from build123d import *

# Parameters (mm, degrees)
EXTRUDE_1_DEPTH     = 40
EXTRUDE_START       = 1
EXTRUDE_2_DEPTH     = 1
CUT_EXTRUDE_7_REACH = 83
FILLET_1_R          = 3
EXTRUDE_6_DEPTH     = 41
SKETCH_2_W          = 15.763743406
SKETCH_2_H          = 16
CUT_EXTRUDE_1_DEPTH = 80
FILLET_2_R          = 1


with BuildPart() as part:
    # 草图1 → 凸台-拉伸1 (new, symmetric)
    with BuildSketch(Plane.XY):
        with BuildLine():
            Line((0, 0), (0, -60))
            ThreePointArc((0, -60), (6, -66), (12, -60))
            Line((12, -60), (12, 0))
            Line((12, 0), (14, 0))
            Line((14, 0), (14, -60))
            ThreePointArc((14, -60), (6, -68), (-2, -60))
            Line((-2, -60), (-2, 0))
            Line((-2, 0), (0, 0))
        make_face()
    extrude(amount=EXTRUDE_1_DEPTH, both=True)

    # 草图3 → 凸台-拉伸2 (add)
    with BuildSketch(Plane.XY.offset(40).offset(EXTRUDE_START)):
        with BuildLine():
            Line((14, -60), (14, 0))
            Line((14, 0), (-2, 0))
            Line((-2, 0), (-2, -60))
            ThreePointArc((-2, -60), (6, -68), (14, -60))
        make_face()
    extrude_2 = extrude(amount=-EXTRUDE_2_DEPTH)

    # 镜向1: 凸台-拉伸2 across plane
    add(extrude_2.mirror(Plane.XY))

    # 切除-拉伸7: up to this face of the body (flat: up to its plane)
    cut_extrude_7_end = Plane(part.part.faces().sort_by_distance((14, -30, 0))[0])
    # 草图4 → 切除-拉伸7 (cut, up to the picked face)
    with BuildSketch(Plane.ZY.offset(2), mode=Mode.PRIVATE) as cut_extrude_7_sk1:
        Polygon((15, -60), (41, -60), (41, -14.966679003), align=None)
    cut_extrude_7_tool1 = split(extrude(cut_extrude_7_sk1.sketch, amount=-CUT_EXTRUDE_7_REACH, mode=Mode.PRIVATE), bisect_by=cut_extrude_7_end, keep=Keep.BOTH, mode=Mode.PRIVATE)
    # 草图4 → 切除-拉伸7 (cut, up to the picked face)
    with BuildSketch(Plane.ZY.offset(2), mode=Mode.PRIVATE) as cut_extrude_7_sk2:
        Polygon((-41, -14.966679003), (-15, -60), (-41, -60), align=None)
    cut_extrude_7_tool2 = split(extrude(cut_extrude_7_sk2.sketch, amount=-CUT_EXTRUDE_7_REACH, mode=Mode.PRIVATE), bisect_by=cut_extrude_7_end, keep=Keep.BOTH, mode=Mode.PRIVATE)
    add(cut_extrude_7_tool1.solids().sort_by(Axis((-2, -44.988893, 32.333333), (1, 0, 0)))[0], mode=Mode.SUBTRACT)
    add(cut_extrude_7_tool2.solids().sort_by(Axis((-2, -44.988893, -32.333333), (1, 0, 0)))[0], mode=Mode.SUBTRACT)

    # 圆角1
    fillet_1_edges = [part.edges().sort_by_distance(p)[0] for p in [
        (13, -60, 15),
        (-1, -60, 15),
        (13, -60, -15),
        (-1, -60, -15),
    ]]
    fillet(fillet_1_edges, radius=FILLET_1_R)

    # 草图7 → 凸台-拉伸6 (add, symmetric)
    with BuildSketch(Plane.XY):
        with BuildLine():
            Line((0.255437353, -64), (-0.92820323, -64))
            Line((-0.92820323, -64), (1.381197846, -68))
            Line((1.381197846, -68), (2.144974753, -68))
            Line((2.144974753, -68), (9.855025247, -68))
            Line((9.855025247, -68), (10.618802154, -68))
            Line((10.618802154, -68), (12.92820323, -64))
            Line((12.92820323, -64), (11.744562647, -64))
            ThreePointArc((11.744562647, -64), (6, -67), (0.255437353, -64))
        make_face()
    extrude(amount=EXTRUDE_6_DEPTH, both=True)

    # 草图2 → 切除-拉伸1 (cut)
    with BuildSketch(Plane(origin=(0, 0, 0), x_dir=(1, 0, 0), z_dir=(0, 1, 0))):
        with Locations((7.881871703, 0)):
            Rectangle(SKETCH_2_W, SKETCH_2_H)
    extrude(amount=-CUT_EXTRUDE_1_DEPTH, mode=Mode.SUBTRACT)

    # 圆角2
    fillet_2_edges = [part.edges().sort_by_distance(p)[0] for p in [
        (12, -8.349364905, 40),
        (-2, -7.483339502, 41),
        (-2, -7.483339502, -41),
        (0, -8.349364905, -40),
        (14, -7.483339502, -41),
        (14, -7.483339502, 41),
        (0, -8.349364905, 40),
        (12, -8.349364905, -40),
    ]]
    fillet(fillet_2_edges, radius=FILLET_2_R)


solid = part.part
The listing builds one solid part. Answer for the finished solid, in the listing's coordinates (mm). A direction names the side the tool comes from. Coordinates: 2 decimals unless noted, no trailing zeros. Write each loop counter-clockwise with the first axis right and the second up, starting at its lowest first coordinate (ties: lowest second). Pieces come first, ordered by that corner, then holes. Notation, with made-up numbers: M -16.75,-2.5 L -11.75,-2.5 A17 ccw -11.75,1.5 Z; hole C 59.5,21 d4. An arc over 180 degrees is marked long. Put each result on its own line as item: value. Start each with the question number.
1. For a pull along X with two mould halves and no side action, classify faces 1 (the flat face through (12.5, -60, -32.1)), 2 (the flat face through (-2, -23, -1)), 3 (the flat face through (6, -62, -40)), 4 (the cylindrical face through (13.72, -62.1, -24.73)) as pulls with the +X half, pulls with the -X half, needs draft (parallel to the pull), parting line crosses it, or undercut.
2. A cutting plane is placed at D-D on z = 12. Write down the section's boundary in (x, y), then the cut area to 3 significant figures.
3. A cutting plane is placed at A-A on x = 6. Write down the section's boundary in (y, z).
4. Flat-ended cylindrical pins translate along their axes: P1, Ø4, axis at x = 5.5, z = 5, coming from the +Y side; P2, Ø7, axis at x = 7.5, y = -18.5, coming from the -Z side. Find the tip coordinate at first contact, or state that the pin passes through.
5. Consider line 1 (X direction, y = -19.5, z = -26); line 2 (Z direction, x = 9.75, y = -6); line 3 (Y direction, x = -0.25, z = 23.5). Determine where each line is inside the solid, lowest interval first. Write a range as from..to.
6. A cutting plane is placed at C-C on y = -41. Write down the section's boundary in (x, z).
7. A cutting plane is placed at B-B on z = -27. Write down the section's boundary in (x, y), then the cut area to 3 significant figures.
8. Which of the six approach directions +Z, -Z, +X, -X, +Y, -Y give full straight-line access (tool end or side, diameter ignored) to faces 5 (the flat face through (6, -8, -40)), 6 (the flat face through (12.48, -33.64, 30.22)), 7 (the flat face through (12.2, -38.9, -8))?
Resolved:
1. face 1: needs draft
1. face 2: pulls with the -X half
1. face 3: undercut
1. face 4: pulls with the +X half
2. outline: M -2,-60 A8 ccw -0.93,-64 L 1.38,-68 L 10.62,-68 L 12.93,-64 A8 ccw 14,-60 L 14,0 L 12,0 L 12,-60 A6 cw 0,-60 L 0,0 L -2,0 Z
2. area: 291 mm2
3. outline: M -68,-41 L -60,-41 L -60,-40 L -66,-40 L -66,-8 L -68,-8 Z; M -68,8 L -66,8 L -66,40 L -60,40 L -60,41 L -68,41 Z; M -16.7,-40 L -14.97,-41 L 0,-41 L 0,-40 Z; M -16.7,40 L 0,40 L 0,41 L -14.97,41 Z
4. P1: passes through
4. P2: stops at z = -40.98
5. line 1: x = -2..0, 12..14
5. line 2: z = -41..-40, 40..41
5. line 3: y = -65.17..-60, -45.28..0
6. outline: M -2,-25.97 L 0,-25.97 L 0,25.97 L -2,25.97 Z; M 12,-25.97 L 14,-25.97 L 14,-8 L 12,-8 Z; M 12,8 L 14,8 L 14,25.97 L 12,25.97 Z
7. outline: M -2,-60 A8 ccw -0.93,-64 L 1.38,-68 L 10.62,-68 L 12.93,-64 A8 ccw 14,-60 L 12,-60 A6 cw 0,-60 Z; M -2,-39.22 L 0,-39.22 L 0,0 L -2,0 Z; M 12,-39.22 L 14,-39.22 L 14,0 L 12,0 Z
7. area: 208 mm2
8. face 5: +Y
8. face 6: +Z, +X, -X
8. face 7: +X, +Y, -Y
